from build123d import *

# Parameters (mm, degrees)
SKETCH1_R               = 1.5
SKETCH1_R_2             = 1
SKETCH1_R_3             = 7
SKETCH1_R_4             = 4.75
BOSS_EXTRUDE1_DEPTH     = 3
CUT_EXTRUDE1_DEPTH      = 179.582042719
CUT_EXTRUDE1_DEPTH_BACK = 179.582042719
SKETCH2_R               = 6.5


with BuildPart() as part:
    # Sketch1 → Boss-Extrude1 (new body)
    with BuildSketch(Plane(origin=(0, 0, 0), x_dir=(0, 0, -1), z_dir=(1, 0, 0))):
        with BuildLine():
            Line((-48.375, 0), (48.375, 0))
            ThreePointArc((48.375, 0), (67.125, 18.75), (48.375, 37.5))
            Line((48.375, 37.5), (40.375, 37.5))
            ThreePointArc((40.375, 37.5), (35.295765254, 38.742880835), (31.364327513, 42.1906592))
            ThreePointArc((31.364327513, 42.1906592), (-27.467628368, 101.587088748), (-102.722095146, 138))
            ThreePointArc((-102.722095146, 138), (-113.291936406, 127.38864025), (-103.88918697, 115.730561375))
            ThreePointArc((-103.88918697, 115.730561375), (-50.193524878, 91.468412174), (-15.975, 43.5))
            ThreePointArc((-15.975, 43.5), (-20.221951673, 33.246951673), (-30.475, 29))
            Line((-30.475, 29), (-48.375, 29))
            ThreePointArc((-48.375, 29), (-62.875, 14.5), (-48.375, 0))
        make_face()
        with Locations((59.625, 18.75)):
            Circle(SKETCH1_R, mode=Mode.SUBTRACT)
        with Locations((54.625, 28.75)):
            Circle(SKETCH1_R_2, mode=Mode.SUBTRACT)
        with Locations((-47.875, 14.5)):
            Circle(SKETCH1_R_3, mode=Mode.SUBTRACT)
        with Locations((-103.305641058, 126.865280687)):
            Circle(SKETCH1_R_4, mode=Mode.SUBTRACT)
        with BuildLine():
            Line((46.625, 23.25), (48.625, 23.25))
            ThreePointArc((48.625, 23.25), (53.125, 18.75), (48.625, 14.25))
            Line((48.625, 14.25), (46.625, 14.25))
            ThreePointArc((46.625, 14.25), (42.125, 18.75), (46.625, 23.25))
        make_face(mode=Mode.SUBTRACT)
        with BuildLine():
            Line((-84.112179989, 120.210043762), (-78.004177954, 117.98691283))
            ThreePointArc((-78.004177954, 117.98691283), (-76.659414879, 115.103059111), (-79.543268599, 113.758296037))
            Line((-79.543268599, 113.758296037), (-85.651270634, 115.981426968))
            ThreePointArc((-85.651270634, 115.981426968), (-86.996033708, 118.865280687), (-84.112179989, 120.210043762))
        make_face(mode=Mode.SUBTRACT)
        with BuildLine():
            Line((-75.120324234, 124.438660555), (-69.012322199, 122.215529624))
            ThreePointArc((-69.012322199, 122.215529624), (-67.667559125, 119.331675904), (-70.551412844, 117.98691283))
            Line((-70.551412844, 117.98691283), (-76.659414879, 120.210043762))
            ThreePointArc((-76.659414879, 120.210043762), (-78.004177954, 123.093897481), (-75.120324234, 124.438660555))
        make_face(mode=Mode.SUBTRACT)
    extrude(amount=BOSS_EXTRUDE1_DEPTH)

    # Sketch2 → Cut-Extrude1 (cut, two sides: drawn at the far end of the back side and taken through both)
    with BuildSketch(Plane(origin=(3, 0, 0), x_dir=(0, 0, -1), z_dir=(1, 0, 0)).offset(-CUT_EXTRUDE1_DEPTH_BACK)):
        with Locations((48.625, 18.75)):
            Circle(SKETCH2_R)
    extrude(amount=CUT_EXTRUDE1_DEPTH + CUT_EXTRUDE1_DEPTH_BACK, mode=Mode.SUBTRACT)


solid = part.part
Here's how the part is built. I have some questions about the finished solid (model axes, mm). A direction names the side the tool comes from. Round coordinates to 2 decimals unless told otherwise and drop trailing zeros. Loops run counter-clockwise (first coordinate to the right, second up) from the corner with the lowest first, then second, coordinate; pieces in that order, holes last. Notation, with made-up numbers: (15.25, -4) -> (39.25, -4) arc R20 ccw to (39.25, 23) -> close; hole circle Ø11 at (39, 86.5). An arc over 180 degrees is marked (long way). Write each question's results on one line, items separated by ' | '.
(1) For faces 4 (the face through (0, 54, 10)), 5 (the face through (1.479, 91.996, 50.84)), which set-ups out of +Z, -Z, +X, -X, +Y, -Y let a thin tool reach every point of the face, with its end or its side?
Worked answers:
face 4: +Z, -Z, -X, +Y, -Y | face 5: +Z, +X, -X
(2) If we section it at D-D, the plane z = 58.5: List the corners of the cut face in (x, y) for me, then the cut area to 3 significant figures.
Worked answers:
outline: (0, 4.12) -> (3, 4.12) -> (3, 24.88) -> (0, 24.88) -> close; (0, 97.68) -> (3, 97.68) -> (3, 120.48) -> (0, 120.48) -> close | area: 131 mm2
(3) If I drill on L1, parallel to Z at x = 0.3, y = 18; L2, parallel to Z at x = 0.4, y = 13; L3, parallel to Y at x = 0.25, z = -40.5, over which ranges is the centre line in solid material (lowest first)?
Worked answers:
L1: -67.11 to -60.92, -58.33 to -55.08, -42.17 to 41.81, 53.94 to 62.45 | L2: -66.22 to -51.66, -45.59 to 41.04, 54.71 to 62.8 | L3: 0 to 37.5
(4) If we section it at C-C, the plane x = 2.55: List the corners of the cut face in (y, z) for me (3 decimals).
Worked answers:
outline: (0, -48.375) arc R18.75 ccw to (37.5, -48.375) -> (37.5, -40.375) arc R11 cw to (42.191, -31.364) arc R247.422 ccw to (138, 102.722) arc R11.216 ccw to (115.731, 103.889) arc R113.159 cw to (43.5, 15.975) arc R14.5 cw to (29, 30.475) -> (29, 48.375) arc R14.5 ccw to (0, 48.375) -> close; hole circle Ø14 at (14.5, 47.875); hole circle Ø13 at (18.75, -48.625); hole circle Ø3 at (18.75, -59.625); hole circle Ø2 at (28.75, -54.625); hole (113.758, 79.543) arc R2.25 ccw to (117.987, 78.004) -> (120.21, 84.112) arc R2.25 ccw to (115.981, 85.651) -> close; hole (117.987, 70.551) arc R2.25 ccw to (122.216, 69.012) -> (124.439, 75.12) arc R2.25 ccw to (120.21, 76.659) -> close; hole circle Ø9.5 at (126.865, 103.306)
(5) We'd pull the mould along Y, two halves only. Please class faces 1 (the face through (1.479, 8.29, 44.645)), 2 (the face through (1.479, 127.618, 113.278)), 3 (the face through (1.48, 100.9, 26.51)): released by +Y, released by -Y, zero draft, split by the parting line, or undercut.
Worked answers:
face 1: undercut | face 2: split by the parting line | face 3: released by +Y
(6) If we section it at B-B, the plane y = 14.5: List the corners of the cut face in (x, z) for me (3 decimals).
Worked answers:
outline: (0, -66.637) -> (3, -66.637) -> (3, -53.543) -> (0, -53.543) -> close; (0, -43.707) -> (3, -43.707) -> (3, 40.875) -> (0, 40.875) -> close; (0, 54.875) -> (3, 54.875) -> (3, 62.875) -> (0, 62.875) -> close
(7) For P1, Ø10, axis at y = 121, z = 89.5, coming from the -X side, with a flat end and sliding along its axis, tell me the tip position at first contact or that it passes through.
Worked answers:
P1: x = 0
(8) If we section it at A-A, the plane z = 26: List the corners of the cut face in (x, y) for me.
Worked answers:
outline: (0, 0) -> (3, 0) -> (3, 29.71) -> (0, 29.71) -> close; (0, 63.9) -> (3, 63.9) -> (3, 100.53) -> (0, 100.53) -> close
